Here's the drawing with two shaded views (mm, measured from the low corner). I have some questions. A direction names the side the tool comes from. Round coordinates to 2 decimals unless told otherwise and drop trailing zeros. Loops run counter-clockwise (first coordinate to the right, second up) from the corner with the lowest first, then second, coordinate; pieces in that order, holes last. Notation, with made-up numbers: M -5,-4 L 39,-4 A24 ccw 39,6 Z; hole C 54.5,20 d7. An arc over 180 degrees is marked long. Answer as a JSON object with one key per item and string values.
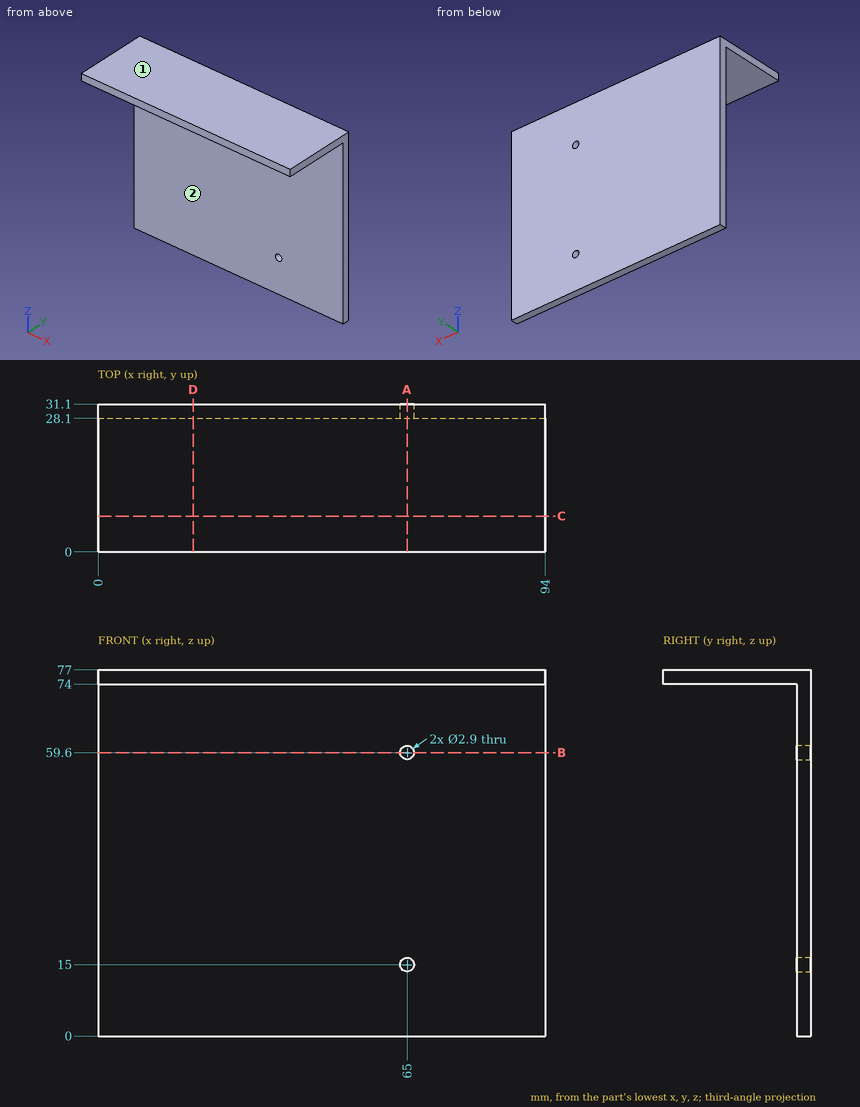
Item 1: I want a section at D-D on x = 20. List the corners of the cut face in (y, z) for me.
Solution:
{"outline": "M 0,74 L 28.1,74 L 28.1,0 L 31.1,0 L 31.1,77 L 0,77 Z"}
Item 2: I want a section at A-A on x = 65. List the corners of the cut face in (y, z) for me.
Solution:
{"outline": "M 0,74 L 28.1,74 L 28.1,61.05 L 31.1,61.05 L 31.1,77 L 0,77 Z; M 28.1,0 L 31.1,0 L 31.1,13.55 L 28.1,13.55 Z; M 28.1,16.45 L 31.1,16.45 L 31.1,58.15 L 28.1,58.15 Z"}
Item 3: If I drill on L1, parallel to Z at x = 65, y = 28.9; L2, parallel to X at y = 29, z = 15; L3, parallel to Z at x = 81, y = 4, over which ranges is the centre line in solid material (lowest first)? Write a range as from..to.
Solution:
{"L1": "z = 0..13.55, 16.45..58.15, 61.05..77", "L2": "x = 0..63.55, 66.45..94", "L3": "z = 74..77"}
Item 4: I want a section at B-B on z = 59.6. List the corners of the cut face in (x, y) for me.
Solution:
{"outline": "M 0,28.1 L 63.55,28.1 L 63.55,31.1 L 0,31.1 Z; M 66.45,28.1 L 94,28.1 L 94,31.1 L 66.45,31.1 Z"}
Item 5: For the marked faces 1 and 2, which set-ups out of +Z, -Z, +X, -X, +Y, -Y let a thin tool reach every point of the face, with its end or its side?
Solution:
{"face 1": "+Z, +X, -X, +Y, -Y", "face 2": "-Z, +X, -X, -Y"}
Item 6: I want a section at C-C on y = 7.5. List the corners of the cut face in (x, z) for me.
Solution:
{"outline": "M 0,74 L 94,74 L 94,77 L 0,77 Z"}
Item 7: For P1, Ø10, axis at y = 27.5, z = 47.5, coming from the +X side, with a flat end and sliding along its axis, tell me the tip position at first contact or that it passes through.
Solution:
{"P1": "stops at x = 94"}
